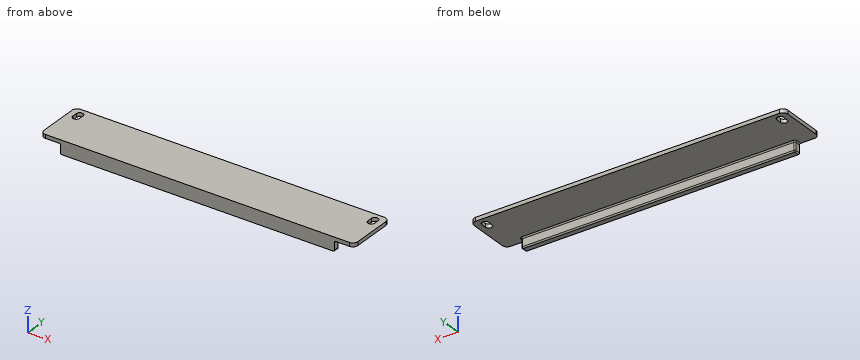
from build123d import *

# Parameters (mm, degrees)
SKETCH1_W           = 252
SKETCH1_H           = 40
BOSS_EXTRUDE1_DEPTH = 3
SKETCH2_W           = 220
SKETCH2_H           = 8
BOSS_EXTRUDE2_DEPTH = 5
FILLET1_R           = 4
FILLET2_R           = 1


with BuildPart() as part:
    # Sketch1 → Boss-Extrude1 (new body)
    with BuildSketch(Plane.XY):
        with Locations((126, 20)):
            Rectangle(SKETCH1_W, SKETCH1_H)
        with BuildLine():
            Line((10.2, 34), (10.2, 30))
            ThreePointArc((10.2, 30), (7.5, 27.3), (4.8, 30))
            Line((4.8, 30), (4.8, 34))
            ThreePointArc((4.8, 34), (7.5, 36.7), (10.2, 34))
        make_face(mode=Mode.SUBTRACT)
        with BuildLine():
            Line((247.2, 34), (247.2, 30))
            ThreePointArc((247.2, 30), (244.5, 27.3), (241.8, 30))
            Line((241.8, 30), (241.8, 34))
            ThreePointArc((241.8, 34), (244.5, 36.7), (247.2, 34))
        make_face(mode=Mode.SUBTRACT)
    extrude(amount=BOSS_EXTRUDE1_DEPTH)

    # Sketch2 → Boss-Extrude2 (add)
    with BuildSketch(Plane.XZ):
        with Locations((126, -4)):
            Rectangle(SKETCH2_W, SKETCH2_H)
    extrude(amount=-BOSS_EXTRUDE2_DEPTH)

    # Fillet1
    fillet1_edges = [part.edges().sort_by_distance(p)[0] for p in [
        (0, 40, 1.5),
        (252, 40, 1.5),
        (252, 0, 1.5),
        (0, 0, 1.5),
    ]]
    fillet(fillet1_edges, radius=FILLET1_R)

    # Fillet2
    fillet2_edges = [part.edges().sort_by_distance(p)[0] for p in [
        (126, 5, 0),
        (16, 2.5, 0),
        (236, 5, -4),
        (236, 2.5, 0),
        (126, 5, -8),
        (236, 2.5, -8),
        (16, 5, -4),
        (16, 2.5, -8),
    ]]
    fillet(fillet2_edges, radius=FILLET2_R)


solid = part.part
Work out the finished part from the listing and answer in its coordinate system (mm). Coordinates: 2 decimals unless noted, no trailing zeros. Loops run counter-clockwise (first coordinate to the right, second up) from the corner with the lowest first, then second, coordinate; pieces in that order, holes last. Notation, with made-up numbers: (46.25, 77.25) -> (94.25, 77.25) arc R22 ccw to (94.25, 100.25) -> close; hole circle Ø10 at (55, -11.5). An arc over 180 degrees is marked (long way). Answer as CSV lines item,"result".
1) The part is cut by section C-C (x = 22.5). Give the vertices of the cut face in (y, z), and give its area (3 significant figures).
A:
outline,"(0, -8) -> (4, -8) arc R1 ccw to (5, -7) -> (5, -1) arc R1 cw to (6, 0) -> (40, 0) -> (40, 3) -> (0, 3) -> close"
area,"160 mm²"
2) The part is cut by section B-B (z = -5). Give the vertices of the cut face in (x, y).
A:
outline,"(16, 0) -> (236, 0) -> (236, 4) arc R1 ccw to (235, 5) -> (17, 5) arc R1 ccw to (16, 4) -> close"
3) Flat-ended cylindrical pins translate along their axes: pin 1 (1 mm diameter, centred on x = 210, z = -3.5, fed in from +Y); pin 2 (3 mm diameter, centred on y = 3, z = -4, fed in from -X); pin 3 (4 mm diameter, centred on x = 158, y = 33, fed in from -Z); pin 4 (1.5 mm diameter, centred on x = 76, z = -2, fed in from -Y). Find the tip coordinate at first contact, or state that the pin passes through.
A:
pin 1,"stops at y = 5"
pin 2,"stops at x = 16"
pin 3,"stops at z = 0"
pin 4,"stops at y = 0"
4) The part is cut by section A-A (x = 244.5). Give the vertices of the cut face in (y, z), and give its area (3 significant figures).
A:
outline,"(0, 0) -> (27.3, 0) -> (27.3, 3) -> (0, 3) -> close; (36.7, 0) -> (40, 0) -> (40, 3) -> (36.7, 3) -> close"
area,"91.8 mm²"
5) The part is cut by section D-D (y = 13). Give the vertices of the cut face in (x, z).
A:
outline,"(0, 0) -> (252, 0) -> (252, 3) -> (0, 3) -> close"
6) Straight lines are drawn through the part: probe 1 along Y at (x, z) = (81.5, -2); probe 2 along Z at (x, y) = (137.5, 20); probe 3 along Y at (x, z) = (164, -7.5). For each, find the intervals that lie inside material, in ascending order.
A:
probe 1,"y = 0 to 5"
probe 2,"z = 0 to 3"
probe 3,"y = 0 to 4.87"
